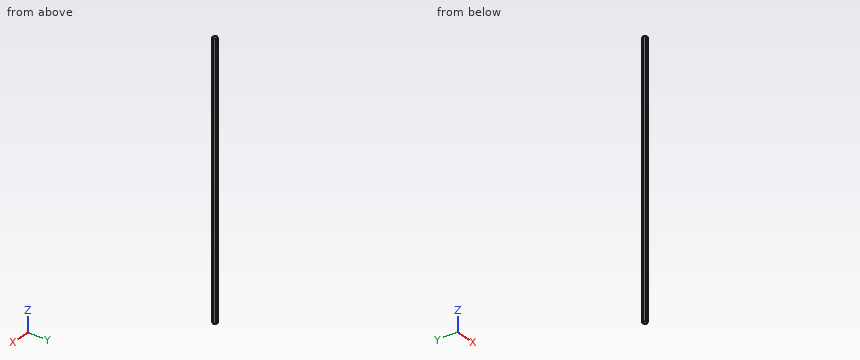
Autodesk Inventor part; units mm, degrees
ref_plane "YZ Plane" through (0, 0, 0) normal (1, 0, 0) x (0, 1, 0)
ref_plane "XZ Plane" through (0, 0, 0) normal (0, 1, 0) x (-1, 0, 0)
ref_plane "XY Plane" through (0, 0, 0) normal (0, 0, 1) x (1, 0, 0)
sketch "Sketch1" plane through (0, 0, 0) normal (0, 0, 1) x (1, 0, 0)
  line L0 (3.6662, 6.35) -> (7.3323, 0)
  line L1 (7.3323, 0) -> (3.6662, -6.35)
  line L2 (3.6662, -6.35) -> (-3.6662, -6.35)
  line L3 (-3.6662, -6.35) -> (-7.3323, 0)
  line L4 (-7.3323, 0) -> (-3.6662, 6.35)
  line L5 (-3.6662, 6.35) -> (3.6662, 6.35)
  point P0 (0, 0)
  dimension "d0" = 12.7
  dimension "d1" = 12.7
extrude "Extrusion1" add sketch "Sketch1" along normal blind 838.2
properties part number "33 in hex shaft"
Can you work these out from the model? Positions are in its coordinate system, mm. Coordinates: 2 decimals unless noted, no trailing zeros. Loops run counter-clockwise (first coordinate to the right, second up) from the corner with the lowest first, then second, coordinate; pieces in that order, holes last.
1) Imagine slicing it at A-A on z = 512. List the corners of the cut face in (x, y) for me.
2) Imagine slicing it at B-B on y = 3.5. List the corners of the cut face in (x, z) for me, plus the area to 3 significant figures.
3) I need wall thicknesses on probe 1 along X at (y, z) = (-1.75, 466.5); probe 2 along Y at (x, z) = (3.75, 448.5); probe 3 along X at (y, z) = (1.5, 767). Which ranges of each line are inside material? Lowest first, please.
Completed:
1. outline: (-7.33, 0) - (-3.67, -6.35) - (3.67, -6.35) - (7.33, 0) - (3.67, 6.35) - (-3.67, 6.35) - close
2. outline: (-5.31, 0) - (5.31, 0) - (5.31, 838.2) - (-5.31, 838.2) - close
2. area: 8,900 mm2
3. probe 1: x = -6.32 to 6.32
3. probe 2: y = -6.2 to 6.2
3. probe 3: x = -6.47 to 6.47
